Autodesk Inventor part; units mm, degrees
ref_plane "YZ Plane" through (0, 0, 0) normal (1, 0, 0) x (0, 1, 0)
ref_plane "XZ Plane" through (0, 0, 0) normal (0, 1, 0) x (-1, 0, 0)
ref_plane "XY Plane" through (0, 0, 0) normal (0, 0, 1) x (1, 0, 0)
sketch "Sketch1" plane through (0, 0, 0) normal (0, 0, 1) x (1, 0, 0)
  line L0 (0, 26.162) -> (0, -85.852)
  line L1 (-192.024, 0) -> (192.024, 0)
  line L2 (137.16, 10.16) -> (-137.16, 10.16)
  line L3 (-137.16, 10.16) -> (-137.16, 0)
  line L4 (-137.16, 0) -> (137.16, 0)
  line L5 (137.16, 0) -> (137.16, 10.16)
  line L6 (137.16, 10.16) -> (-137.16, 0) construction
  line L7 (-137.16, 10.16) -> (137.16, 0) construction
  line L8 (62.865, -69.85) -> (-62.865, -69.85)
  line L9 (-62.865, -69.85) -> (-62.865, 0)
  line L10 (-62.865, 0) -> (62.865, 0)
  line L11 (62.865, 0) -> (62.865, -69.85)
  line L12 (62.865, -69.85) -> (-62.865, 0) construction
  line L13 (-62.865, -69.85) -> (62.865, 0) construction
  point P0 (0, 0)
  point P1 (0, 5.08)
  point P2 (0, 5.588)
  point P3 (-132.08, 5.588)
  point P4 (132.08, 5.588)
  point P5 (0, -34.925)
  point P6 (12.7, -31.75)
  point P7 (-38.1, 5.588)
  point P8 (38.1, 5.588)
  point P9 (-50.8, -59.69)
  point P10 (50.8, -59.69)
  point P11 (0, -34.925)
  dimension "d0" = 274.32
  dimension "d1" = 10.16
  dimension "d2" = 5.588
  dimension "d13" = 5.08
  dimension "d14" = 5.08
  dimension "d15" = 69.85
  dimension "d16" = 125.73
  dimension "d29" = 38.1
  dimension "d30" = 38.1
  dimension "d31" = 101.6
  dimension "d32" = 50.8
  dimension "d33" = 10.16
  dimension "d44" = 31.75
  dimension "d45" = 12.7
extrude "Extrusion1" add sketch "Sketch1" against normal blind 4.4958 contours L2 L5 L1 L0 | L0 L1 L3 L2
hole "Hole1" at (0, 5.588, 0) at (-132.08, 5.588, 0) at (132.08, 5.588, 0) at (-38.1, 5.588, 0) at (38.1, 5.588, 0) direction (0, 0, -1) diameter 3.81 end through all
fillet "Fillet1" radius 3.175 2 edges at (-137.16, 10.16, -2.2479) (137.16, 10.16, -2.2479)
extrude "Extrusion2" add sketch "Sketch1" against normal up to surface (4.4958 mm away) contours L1 L11 L8 L0 | L0 L8 L9 L1
fillet "Fillet2" radius 9.525 2 edges at (-62.865, -69.85, -2.2479) (62.865, -69.85, -2.2479)
hole "Hole2" at (12.7, -31.75, 0) direction (0, 0, -1) diameter 3.3528 end through all
hole "Hole3" at (-50.8, -59.69, 0) at (50.8, -59.69, 0) direction (0, 0, -1) diameter 3.81 end through all
pattern_linear "Rectangular Pattern1" count 4 spacing 9.525 along (0, -1, 0) count 2 spacing 25.4 along (-1, 0, 0) of "Hole2"
Can you work these out from the model? Positions are in its coordinate system, mm. A direction names the side the tool comes from. Round coordinates to 2 decimals unless told otherwise and drop trailing zeros. Loops run counter-clockwise (first coordinate to the right, second up) from the corner with the lowest first, then second, coordinate; pieces in that order, holes last. Notation, with made-up numbers: (6, -29.75) -> (32, -29.75) arc R22 cw to (32, -16.75) -> close; hole circle Ø5 at (87, -35.75). An arc over 180 degrees is marked (long way). Answer in a Markdown table with one row per item.
Item 1: If I drill on probe 1 along X at (y, z) = (-51, -3.8) (3 decimals); probe 2 along Y at (x, z) = (12.7, -1.25); probe 3 along X at (y, z) = (-60.5, -3.55), over which ranges is the centre line in solid material (lowest first)?
Answer block:
| item | result |
|---|---|
| probe 1 | -62.865 to -14.364, -11.036 to 11.036, 14.364 to 62.865 |
| probe 2 | -69.85 to -62, -58.65 to -52.48, -49.12 to -42.95, -39.6 to -33.43, -30.07 to 10.16 |
| probe 3 | -62.86 to -52.52, -49.08 to -14.37, -11.03 to 11.03, 14.37 to 49.08, 52.52 to 62.86 |
Item 2: On a 3-axis mill with a long thin cutter (end or side, diameter ignored), from which of +Z, -Z, +X, -X, +Y, -Y can I reach the whole of each face in a straight line? I mean faces 1 (the flat face through (-2, -29, 0)), 2 (the flat face through (62.865, -30, -2)), 3 (the flat face through (-101, 0, -2)). Say none if no direction works.
Answer block:
| item | result |
|---|---|
| face 1 | +Z, +X, -X, +Y, -Y |
| face 2 | +Z, -Z, +X, -Y |
| face 3 | +Z, -Z, -X, -Y |
Item 3: Will these pins go through, and if not, where does the flat tip stop? P1, Ø2, axis at y = -41, z = -2, coming from the -X side (3 decimals); P2, Ø1.3, axis at y = -37.5, z = -3, coming from the +X side (3 decimals).
Answer block:
| item | result |
|---|---|
| P1 | x = -62.865 |
| P2 | x = 62.865 |
Item 4: Suppose I cut it at B-B, the plane x = 106. List the corners of the cut face in (y, z) for me, plus the area to 3 significant figures.
Answer block:
| item | result |
|---|---|
| outline | (0, -4.5) -> (10.16, -4.5) -> (10.16, 0) -> (0, 0) -> close |
| area | 45.7 mm² |
Item 5: Suppose I cut it at A-A, the plane z = -0.7. Give the number of separate pieces and of enclosed holes in the cut face, plus the area to 3 significant figures.
Answer block:
| item | result |
|---|---|
| separate pieces | 1 |
| enclosed holes | 15 |
| area | 11,400 mm² |
